Autodesk Inventor part; units mm, degrees
ref_plane "YZ Plane" through (0, 0, 0) normal (1, 0, 0) x (0, 1, 0)
ref_plane "XZ Plane" through (0, 0, 0) normal (0, 1, 0) x (-1, 0, 0)
ref_plane "XY Plane" through (0, 0, 0) normal (0, 0, 1) x (1, 0, 0)
sketch "Sketch1" plane through (0, 0, 0) normal (0, 1, 0) x (-1, 0, 0)
  line L0 (15, 20) -> (-15, 20)
  line L1 (-15, 20) -> (-15, -20)
  line L2 (-15, -20) -> (15, -20)
  line L3 (15, -20) -> (15, 20)
  line L4 (15, 20) -> (-15, -20) construction
  line L5 (-15, 20) -> (15, -20) construction
  point P0 (0, 0)
  dimension "d2" = 30
  dimension "d3" = 40
extrude "Extrusion1" add sketch "Sketch1" along normal mid plane 5
sketch "Sketch3" plane through (0, 2.5, 0) normal (0, 1, 0) x (1, 0, 0)
  line L0 (-15, 20) -> (-15, -20)
  line L1 (15, -20) -> (15, 20)
  line L2 (-15, -20) -> (15, -20)
  line L3 (15, 20) -> (-15, 20)
  point P0 (0, 0)
  point P1 (0, -12)
  point P2 (-15, 0)
  dimension "d28" = 8
hole "Hole1" at (0, 2.5, 12) direction (0, -1, 0) diameter 4.305 end through all
sketch "Sketch4" plane through (0, -2.5, 0) normal (0, -1, 0) x (1, 0, 0)
  circle A0 centre (0, -4.477) radius 3.8735
  circle A1 centre (0, 12) radius 2.1525
  point P0 (0, 0)
  dimension "d16" = 7.747
  dimension "d17" = 16.477
extrude "Extrusion3" add sketch "Sketch4" along normal blind 3 contours A0
sketch "Sketch5" plane through (0, -2.5, 0) normal (0, -1, 0) x (1, 0, 0)
  circle A0 centre (10, -14.477) radius 1.5
  line L0 (-15, -20) -> (15, -20)
  line L1 (-15, 20) -> (-15, -20)
  line L2 (15, -20) -> (15, 20)
  circle A1 centre (0, -4.477) radius 3.8735
  circle A2 centre (0, 12) radius 2.1525
  line L3 (15, 20) -> (-15, 20)
  line L4 (-15, 20) -> (-15, -20)
  line L5 (-15, -20) -> (15, -20)
  line L6 (15, -20) -> (15, 20)
  point P0 (0, 0)
  dimension "d20" = 3
  dimension "d33" = 10
  dimension "d34" = 10
extrude "Extrusion4" cut sketch "Sketch5" against normal through all contours A0
sketch "Sketch6" plane through (0, 2.5, 0) normal (0, 1, 0) x (1, 0, 0)
  circle A0 centre (0, -12) radius 2.1525
  circle A1 centre (0, -12) radius 4
  point P0 (0, 0)
  dimension "d30" = 8
extrude "Extrusion5" cut sketch "Sketch6" against normal blind 2
sketch "Sketch7" plane through (0, -2.5, 0) normal (0, -1, 0) x (1, 0, 0)
  line L0 (15, 20) -> (15, -20)
  line L1 (15, 20) -> (-15, 20)
  line L2 (-15, 20) -> (-15, 17)
  line L3 (-15, 17) -> (15, 17)
  line L4 (15, 17) -> (15, 20)
  line L5 (-15, 20) -> (-15, -20)
  point P0 (0, 0)
  dimension "d35" = 3
extrude "Extrusion6" add sketch "Sketch7" along normal blind 2
fillet "Fillet1" radius 2 4 edges at (15, -1, 20) (-15, -1, 20) (15, 0, -20) (-15, 0, -20)
properties part number "PinionHolderTest"
Verification items for the finished model (mm, model axes). A direction names the side the tool comes from. Coordinates: 2 decimals unless noted, no trailing zeros. Write each loop counter-clockwise with the first axis right and the second up, starting at its lowest first coordinate (ties: lowest second). Pieces come first, ordered by that corner, then holes. Notation, with made-up numbers: (-10.75, 42.5) -> (0.25, 42.5) arc R20 cw to (0.25, 67.5) -> close; hole circle Ø11 at (77, 1). An arc over 180 degrees is marked (long way). One line per item, written item: value. Start each with the question number.
Q1. Go/stop test with flat-tipped pins: P1, Ø12, axis at x = 1.5, z = 12.5, coming from the +Y side; P2, Ø1, axis at x = 10, z = -1, coming from the -Y side; P3, Ø2.5, axis at x = 0, z = 18.5, coming from the -Y side; P4, Ø0.6, axis at x = 4.5, y = -4, coming from the -Z side. Record where each tip stops, or that it passes through.
Q2. Thickness scan on L1, parallel to Z at x = 0, y = -1.05; L2, parallel to Z at x = 0, y = 1.95; L3, parallel to Y at x = 3.25, z = -16.5. Record the ranges inside material, lowest first. Write a range as from..to.
Q3. Cross-section at A-A on x = 10. Enter the section's corners in (y, z).
Q4. Access from +Z, -Z, +X, -X, +Y, -Y to the whole of each face (thin tool, end or side, straight path). Record for faces 5 (the flat face through (0, -3, 17)), 6 (the cylindrical face through (-0.84, -3.979, -0.696)), 7 (the flat face through (0, -4.5, 19)).
Q5. Cross-section at C-C on y = -1.5. Enter the section's corners in (x, z) (1 decimal), and give its area (3 significant figures).
Q6. Mould release check, pull along X, two halves, no side actions. Record for faces 1 (the cylindrical face through (-0.867, 1.514, 15.905)), 2 (the cylindrical face through (-14.43, -0.04, -19.4)), 3 (the flat face through (15, 1, 0)), 4 (the flat face through (2, 0.5, 14)): pulls with the +X half, pulls with the -X half, needs draft (parallel to the pull), parting line crosses it, or undercut.
Q7. Cross-section at B-B on z = 12. Enter the section's corners in (x, y).
Q8. Cross-section at D-D on y = -3.75. Enter the section's corners in (x, z).
Checked values:
1. P1: stops at y = 2.5
1. P2: stops at y = -2.5
1. P3: stops at y = -4.5
1. P4: stops at z = 17
2. L1: z = -20..9.85, 14.15..20
2. L2: z = -20..8, 16..20
2. L3: y = -2.5..2.5
3. outline: (-4.5, 17) -> (-2.5, 17) -> (-2.5, -12.98) -> (2.5, -12.98) -> (2.5, 20) -> (-4.5, 20) -> close; (-2.5, -20) -> (2.5, -20) -> (2.5, -15.98) -> (-2.5, -15.98) -> close
4. face 5: +X, -X, -Y
4. face 6: -Y
4. face 7: +Z, +X, -X, -Y
5. outline: (-15, -18) arc R2 ccw to (-13, -20) -> (13, -20) arc R2 ccw to (15, -18) -> (15, 18) arc R2 ccw to (13, 20) -> (-13, 20) arc R2 ccw to (-15, 18) -> close; hole circle Ø4.3 at (0, 12); hole circle Ø3 at (10, -14.5)
5. area: 1,170 mm²
6. face 1: undercut
6. face 2: pulls with the -X half
6. face 3: pulls with the +X half
6. face 4: undercut
7. outline: (-15, -2.5) -> (-2.15, -2.5) -> (-2.15, 0.5) -> (-4, 0.5) -> (-4, 2.5) -> (-15, 2.5) -> close; (2.15, -2.5) -> (15, -2.5) -> (15, 2.5) -> (4, 2.5) -> (4, 0.5) -> (2.15, 0.5) -> close
8. outline: (-15, 17) -> (15, 17) -> (15, 18) arc R2 ccw to (13, 20) -> (-13, 20) arc R2 ccw to (-15, 18) -> close; circle Ø7.75 at (0, -4.48)
